Input: part model. Units: mm. Frame: model coordinates. A direction names the side the tool comes from. Round coordinates to 2 decimals unless told otherwise and drop trailing zeros. Loops run counter-clockwise (first coordinate to the right, second up) from the corner with the lowest first, then second, coordinate; pieces in that order, holes last. Notation, with made-up numbers: M 82,12.5 L 127,12.5 A13 cw 127,26.5 Z; hole C 86.5,29.5 d9. An arc over 180 degrees is marked long. Use one line per item in the form item = value. Start each with the question number.
Q1. Ray query, line 1 along Y through (x, z) = (-0.1, 0.25); line 2 along Z through (x, y) = (1.1, -0.25); line 3 along Y through (x, z) = (0.4, 3). Return the intervals inside material, ascending.
Q2. Access query for faces 1 (the cylindrical face through (-1.5, -0.07, -0.67)), 2 (the cylindrical face through (0, -1, -5)), 3 (the cylindrical face through (0, -1, 4)). Directions: +Z, -Z, +X, -X, +Y, -Y. A direction counts if a zero-diameter tool reaches every point of the face in a straight line with its end or side. Return the directions, or none.
Q3. First-contact query: P1, Ø1, axis at y = 1, z = -2, coming from the -X side. Flat tip, straight axial feed; report the tip coordinate or a pass-through.
Q4. Section query C-C, the plane z = -2.75. Output: boundary loops of the cut face in (x, y).
Q5. Section query A-A, the plane y = 0. Output: boundary loops of the cut face in (x, z), and give its area (3 significant figures).
Autodesk Inventor part; units mm, degrees
sketch "Skizze1" plane through (0, 0, 0) normal (0, 0, 1) x (1, 0, 0)
  circle A0 centre (0, 0) radius 1.5
  dimension "d0" = 3
extrude "Extrusion1" add sketch "Skizze1" along normal mid plane 12
sketch "Skizze2" plane through (0, 0, 6) normal (0, 0, 1) x (1, 0, 0)
  circle A0 centre (0, 0) radius 1
  circle A1 centre (0, 0) radius 1.5
  dimension "d3" = 2
extrude "Extrusion2" cut sketch "Skizze2" against normal blind 3.25
thread "Gewinde2"
fillet "Rundung1" radius 0.25 1 edges at (-1.5, 0, 2.75)
sketch "Skizze3" plane through (0, 0, -6) normal (0, 0, -1) x (-1, 0, 0)
  circle A0 centre (0, 0) radius 1
  circle A1 centre (0, 0) radius 1.5
  dimension "d11" = 2
extrude "Extrusion3" cut sketch "Skizze3" against normal blind 2
thread "Gewinde3"
fillet "Rundung2" radius 0.25 1 edges at (-1.5, 0, -4)
properties part number "SchleppstangeBefestigung"
Results found:
q1.line_1 = -1.5 to 1.5
q1.line_2 = -4 to 2.75
q1.line_3 = -0.92 to 0.92
q2.face_1 = +Z, -Z
q2.face_2 = -Z
q2.face_3 = +Z
q3.P1 = -1.41
q4.outline = C 0,0 d3
q5.outline = M -1.5,-3.75 A0.25 ccw -1.25,-4 L -1,-4 L -1,-6 L 1,-6 L 1,-4 L 1.25,-4 A0.25 ccw 1.5,-3.75 L 1.5,2.5 A0.25 ccw 1.25,2.75 L 1,2.75 L 1,6 L -1,6 L -1,2.75 L -1.25,2.75 A0.25 ccw -1.5,2.5 Z
q5.area = 30.7 mm²
